For this review, take the finished solid that the model builds, in its own axes (mm). A direction names the side the tool comes from. Round coordinates to 2 decimals unless told otherwise and drop trailing zeros. Write each loop counter-clockwise with the first axis right and the second up, starting at its lowest first coordinate (ties: lowest second). Pieces come first, ordered by that corner, then holes. Notation, with made-up numbers: (62, 79.5) -> (97, 79.5) arc R19 cw to (97, 93.5) -> close; hole circle Ø2 at (41, 41). An arc over 180 degrees is marked (long way). Answer as CSV lines item,"result". Start each with the question number.
Item 1: Wall thickness on probe 1 along X at (y, z) = (-5.5, 6.25); probe 2 along Y at (x, z) = (14.5, 0.25); probe 3 along X at (y, z) = (4.75, -9): over which ranges is each line inside the solid? List them lowest first. Write a range as from..to.
Item 2: Machinability: for faces 1 (the flat face through (65, 0, 8)), 2 (the cylindrical face through (64, 0, -10)), 3 (the flat face through (20, 8, 2)), 4 (the flat face through (57, 0, -8)), which of the approach directions +Z, -Z, +X, -X, +Y, -Y give a long, thin tool a straight path to every point of the face, cutting with its end or side? Answer none if there is none.
Item 3: Take a section at B-B on y = 0. Give the boundary of the cut face in (x, z), then the cut area to 3 significant figures.
Item 4: Take a section at D-D on x = 10. Give the boundary of the cut face in (y, z), then the cut area to 3 significant figures.
Item 5: Take a section at C-C on x = 53. Give the boundary of the cut face in (y, z), then the cut area to 3 significant figures.
Item 6: Take a section at A-A on z = 0. Give the boundary of the cut face in (x, y).
Item 7: Mouldability with a two-part tool opening along X and no side actions: class faces 5 (the cylindrical face through (54.465, -0.33, -7.493)), 6 (the flat face through (52, 5, 6)), 7 (the flat face through (72, 0, -1)), 8 (the flat face through (0, 0, 0)) as +X half, -X half, draft (parallel to the pull), parting line (faces both ways), or undercut.
Item 8: For pin 1 Ø1 at (x, z) = (55, 2) entering from +Y; pin 2 Ø8 at (x, z) = (50.5, 7.5) entering from -Y; pin 3 Ø8 at (x, y) = (34.5, -7.5) entering from -Z, all flat-tipped, find the tip position at first contact; note any pin that passes through.
```python
from build123d import *

# Parameters (mm, degrees)
F2_SIZE  = 1
F4_DEPTH = 15


with BuildPart() as f1:
    # F0 (on Front) → F1 (revolve)
    with BuildSketch(Plane.XZ):
        Polygon((0, 8), (0, 0), (72, 0), (72, 10), (57, 10), (57, 7.5), (52, 7.5), (52, 12), (20, 12), (20, 8), align=None)
    revolve(axis=Axis((33.058259, 0, 0), (1, 0, 0)))

    # F2
    f2_edges = [f1.edges().sort_by_distance(p)[0] for p in [
        (0, 0, -8),
    ]]
    chamfer(f2_edges, length=F2_SIZE)

    # F3 (on face) → F4 (cut)
    with BuildSketch(Plane.YZ.offset(72)):
        with BuildLine():
            Line((-6, 8), (6, 8))
            ThreePointArc((6, 8), (0, 10), (-6, 8))
        make_face()
    extrude(amount=-F4_DEPTH, mode=Mode.SUBTRACT)


solid = f1.part
```
Output values:
1,probe 1,"x = 20..52, 57..72"
1,probe 2,"y = -8..8"
1,probe 3,"x = 20..52"
2,face 1,"+Z, +X, +Y, -Y"
2,face 2,"+X"
2,face 3,"-X"
2,face 4,"none"
3,outline,"(0, -7) -> (1, -8) -> (20, -8) -> (20, -12) -> (52, -12) -> (52, -7.5) -> (57, -7.5) -> (57, -10) -> (72, -10) -> (72, 8) -> (57, 8) -> (57, 7.5) -> (52, 7.5) -> (52, 12) -> (20, 12) -> (20, 8) -> (1, 8) -> (0, 7) -> close"
3,area,"1,430 mm^2"
4,outline,"circle Ø16 at (0, 0)"
4,area,"201 mm^2"
5,outline,"circle Ø15 at (0, 0)"
5,area,"177 mm^2"
6,outline,"(0, -7) -> (1, -8) -> (20, -8) -> (20, -12) -> (52, -12) -> (52, -7.5) -> (57, -7.5) -> (57, -10) -> (72, -10) -> (72, 10) -> (57, 10) -> (57, 7.5) -> (52, 7.5) -> (52, 12) -> (20, 12) -> (20, 8) -> (1, 8) -> (0, 7) -> close"
7,face 5,"undercut"
7,face 6,"undercut"
7,face 7,"+X half"
7,face 8,"-X half"
8,pin 1,"stops at y = 7.35"
8,pin 2,"stops at y = -11.48"
8,pin 3,"stops at z = -11.48"
